Verification items for the finished model (mm, model axes). Face numbers are marked on the shaded views. A direction names the side the tool comes from. Coordinates: 2 decimals unless noted, no trailing zeros. Write each loop counter-clockwise with the first axis right and the second up, starting at its lowest first coordinate (ties: lowest second). Pieces come first, ordered by that corner, then holes. Notation, with made-up numbers: (27, 0.5) -> (58, 0.5) arc R32 ccw to (58, 36.5) -> close; hole circle Ø1 at (28, -32). An arc over 180 degrees is marked (long way). Write item = value, one per line. Start each with the question number.
(1) Section check C-C (z = -5). Record the cut outline in (x, y).
(2) Section check A-A (x = 0). Record the cut outline in (y, z) (3 decimals), plus the area to 3 significant figures.
(3) Material ranges on probe 1 along Y at (x, z) = (-3.5, -1.5); probe 2 along X at (y, z) = (6.5, 2.25); probe 3 along X at (y, z) = (8, -3.5), recorded low to high. Write a range as [from, to].
(4) Mould release check, pull along Y, two halves, no side actions. Record for the marked faces 3, 4 and 5: released by +Y, released by -Y, zero draft, split by the parting line, or undercut.
(5) Section check D-D (y = 2.75). Record the cut outline in (x, z), plus the area to 3 significant figures.
(6) Gauge pin test, flat ends, axial feed: pin 1 Ø6 at (y, z) = (8, -7) entering from -X; pin 2 Ø1 at (y, z) = (3, -2.5) entering from +X; pin 3 Ø4 at (x, z) = (-2.5, 6) entering from -Y. Record the tip position at first contact, or that the pin passes through.
(7) Set-up check for the marked faces 1 and 2: record each of +Z, -Z, +X, -X, +Y, -Y from which the full face is reachable in a straight line by a thin tool's end or side.
```python
from build123d import *

# Parameters (mm, degrees)
CUT_EXTRUDE2_DEPTH = 11.1252


with BuildPart() as part:
    # Sketch3 → Revolve1 (revolve)
    with BuildSketch(Plane.XY):
        with BuildLine():
            Line((3.9116, 3.5052), (3.9116, 0.8636))
            Line((3.9116, 0.8636), (3.048, 0))
            Line((3.048, 0), (0, 0))
            Line((0, 0), (0, 11.1252))
            ThreePointArc((0, 11.1252), (5.586411751, 10.629871711), (10.9985175, 9.159341969))
            Line((10.9985175, 9.159341969), (10.9985175, 6.35))
            Line((10.9985175, 6.35), (3.429, 6.35))
            ThreePointArc((3.429, 6.35), (3.159592316, 6.238407684), (3.048, 5.969))
            Line((3.048, 5.969), (3.048, 4.3688))
            Line((3.048, 4.3688), (3.9116, 3.5052))
        make_face()
    revolve(axis=Axis((0, -1000, 0), (0, 1, 0)))

    # Sketch1 → Cut-Extrude2 (cut)
    with BuildSketch(Plane(origin=(0, 0, 0), x_dir=(1, 0, 0), z_dir=(0, 1, 0))):
        with BuildLine():
            ThreePointArc((-5.499261314, -9.525), (0, -10.998522628), (5.499261314, -9.525))
            Line((5.499261314, -9.525), (-5.499261314, -9.525))
        make_face()
        with BuildLine():
            ThreePointArc((-10.998522628, 0), (-9.525, -5.499261314), (-5.499261314, -9.525))
            Line((-5.499261314, -9.525), (-10.998522628, 0))
        make_face()
        with BuildLine():
            ThreePointArc((5.499261314, -9.525), (9.525, -5.499261314), (10.998522628, 0))
            Line((10.998522628, 0), (5.499261314, -9.525))
        make_face()
        with BuildLine():
            Line((5.499261314, 9.525), (10.998522628, 0))
            ThreePointArc((10.998522628, 0), (9.525, 5.499261314), (5.499261314, 9.525))
        make_face()
        with BuildLine():
            Line((-5.499261314, 9.525), (5.499261314, 9.525))
            ThreePointArc((5.499261314, 9.525), (0, 10.998522628), (-5.499261314, 9.525))
        make_face()
        with BuildLine():
            Line((-10.998522628, 0), (-5.499261314, 9.525))
            ThreePointArc((-5.499261314, 9.525), (-9.525, 5.499261314), (-10.998522628, 0))
        make_face()
    extrude(amount=CUT_EXTRUDE2_DEPTH, mode=Mode.SUBTRACT)


solid = part.part
```
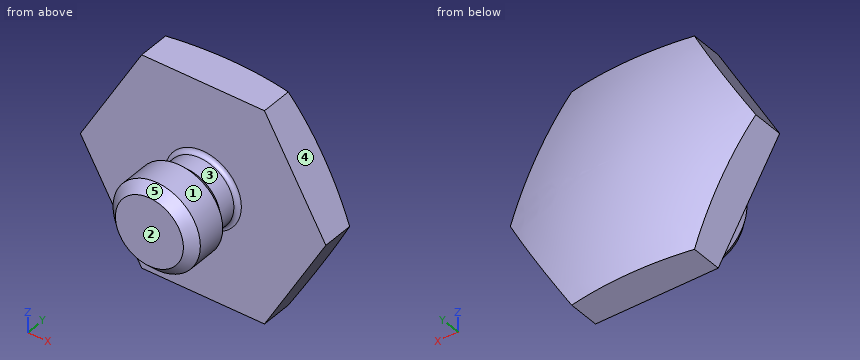
Response:
q1.outline = (-8.11, 6.35) -> (8.11, 6.35) -> (8.11, 9.66) arc R31.35 ccw to (-8.11, 9.66) -> close
q2.outline = (0, -3.048) -> (0.864, -3.912) -> (3.505, -3.912) -> (4.369, -3.048) -> (5.969, -3.048) arc R0.381 cw to (6.35, -3.429) -> (6.35, -9.525) -> (9.663, -9.525) arc R31.75 ccw to (9.663, 9.525) -> (6.35, 9.525) -> (6.35, 3.429) arc R0.381 cw to (5.969, 3.048) -> (4.369, 3.048) -> (3.505, 3.912) -> (0.864, 3.912) -> (0, 3.048) -> close
q2.area = 127 mm2
q3.probe_1 = [0.76, 3.61], [6.35, 10.9]
q3.probe_2 = [-9.7, 9.7]
q3.probe_3 = [-8.98, 8.98]
q4.face_3 = undercut
q4.face_4 = zero draft
q4.face_5 = released by -Y
q5.outline = circle Ø7.82 at (0, 0)
q5.area = 48.1 mm2
q6.pin_1 = -8.69
q6.pin_2 = 3.36
q6.pin_3 = 6.35
q7.face_1 = -Y
q7.face_2 = +Z, -Z, +X, -X, -Y
